```python
from build123d import *

# Parameters (mm, degrees)
F1_DEPTH = 150
F0_W     = 860
F0_H     = 460
F2_DEPTH = 20
F3_DEPTH = 250


with BuildPart() as f1:
    # F0 (on Top) → F1 (new body)
    with BuildSketch(Plane.XY):
        Polygon((430, -230), (450, -230), (450, 230), (450, 250), (-450, 250), (-450, -230), (-430, -230), (-430, 230), (430, 230), align=None)
    extrude(amount=F1_DEPTH)

    # F0 (on Top) → F2 (join)
    with BuildSketch(Plane.XY):
        Polygon((-450, -250), (450, -250), (450, -230), (430, -230), (-430, -230), (-450, -230), align=None)
        Polygon((430, -230), (450, -230), (450, 230), (450, 250), (-450, 250), (-450, -230), (-430, -230), (-430, 230), (430, 230), align=None)
        Rectangle(F0_W, F0_H)
    extrude(amount=F2_DEPTH)

    # F0 (on Top) → F3 (join)
    with BuildSketch(Plane.XY):
        Polygon((-450, -250), (450, -250), (450, -230), (430, -230), (-430, -230), (-450, -230), align=None)
    extrude(amount=F3_DEPTH)


solid = f1.part
```
Input: part model. Units: mm. Frame: model coordinates. A direction names the side the tool comes from. Coordinates: 2 decimals unless noted, no trailing zeros. Loops run counter-clockwise (first coordinate to the right, second up) from the corner with the lowest first, then second, coordinate; pieces in that order, holes last. Notation, with made-up numbers: M 50.25,27 L 83.25,27 A26 cw 83.25,63 Z; hole C 85,49.25 d11. An arc over 180 degrees is marked long. Answer in a Markdown table with one row per item.
1. Reachability of faces 1 (the flat face through (-2, 242, 150)), 2 (the flat face through (6, 250, 74)), 3 (the flat face through (430, 3, 84)) from +Z, -Z, +X, -X, +Y, -Y: full face, straight path, thin tool, end or side. Return the list, or none.
Response:
| item | result |
|---|---|
| face 1 | +Z, +X, -X, +Y |
| face 2 | +Z, -Z, +X, -X, +Y |
| face 3 | +Z |
2. Section A-A, the plane x = -71. Output: boundary loops of the cut face in (y, z), then the cut area to 3 significant figures.
Response:
| item | result |
|---|---|
| outline | M -250,0 L 250,0 L 250,150 L 230,150 L 230,20 L -230,20 L -230,250 L -250,250 Z |
| area | 17,200 mm2 |
3. Section D-D, the plane z = 226.5. Output: boundary loops of the cut face in (x, y), then the cut area to 3 significant figures.
Response:
| item | result |
|---|---|
| outline | M -450,-250 L 450,-250 L 450,-230 L -450,-230 Z |
| area | 18,000 mm2 |
4. Section B-B, the plane z = 122.5. Output: boundary loops of the cut face in (x, y), then the cut area to 3 significant figures.
Response:
| item | result |
|---|---|
| outline | M -450,-250 L 450,-250 L 450,250 L -450,250 Z; hole M -430,-230 L 430,-230 L 430,230 L -430,230 Z |
| area | 54,400 mm2 |
5. First-contact query: pin 1 (8 mm diameter, centred on x = -60.5, z = 215.5, fed in from +Y); pin 2 (6 mm diameter, centred on x = -46, y = -25.5, fed in from +Z). Flat tips, straight axial feed; report the tip coordinate or a pass-through.
Response:
| item | result |
|---|---|
| pin 1 | stops at y = -230 |
| pin 2 | stops at z = 20 |
6. Draft query along X for faces 4 (the flat face through (-6, -240, 250)), 5 (the flat face through (450, -3, 68)), 6 (the flat face through (-450, 3, 68)), 7 (the flat face through (6, -230, 133)). Return one class per face: pulls with the +X half, pulls with the -X half, needs draft (parallel to the pull), parting line crosses it, or undercut.
Response:
| item | result |
|---|---|
| face 4 | needs draft |
| face 5 | pulls with the +X half |
| face 6 | pulls with the -X half |
| face 7 | undercut |
7. Material intervals for line 1 (X direction, y = -139.5, z = 78); line 2 (Y direction, x = -335.5, z = 110); line 3 (Z direction, x = 298, y = -93), sorted ascending.
Response:
| item | result |
|---|---|
| line 1 | x = -450 to -430, 430 to 450 |
| line 2 | y = -250 to -230, 230 to 250 |
| line 3 | z = 0 to 20 |
8. Section C-C, the plane y = 55. Output: boundary loops of the cut face in (x, z), then the cut area to 3 significant figures.
Response:
| item | result |
|---|---|
| outline | M -450,0 L 450,0 L 450,150 L 430,150 L 430,20 L -430,20 L -430,150 L -450,150 Z |
| area | 23,200 mm2 |
